Autodesk Inventor part; units mm, degrees
ref_plane "YZ Plane" through (0, 0, 0) normal (1, 0, 0) x (0, 1, 0)
ref_plane "XZ Plane" through (0, 0, 0) normal (0, 1, 0) x (-1, 0, 0)
ref_plane "XY Plane" through (0, 0, 0) normal (0, 0, 1) x (1, 0, 0)
sketch "Sketch7" plane through (0, 0, 0) normal (0, 1, 0) x (-1, 0, 0)
  circle A0 centre (0, 0) radius 25
  circle A1 centre (0, 0) radius 15
  dimension "d19" = 50
  dimension "d20" = 30
extrude "Extrusion5" add sketch "Sketch7" against normal blind 30 contours A1
extrude "Extrusion6" add sketch "Sketch7" along normal blind 200 contours A0 | A1
sketch "Sketch8" plane through (0, 0, 0) normal (1, 0, 0) x (0, 1, 0)
  line L0 (200, -25) -> (200, 25)
  line L1 (0, -25) -> (0, 25)
  line L2 (0, 25) -> (200, 25)
  line L3 (0, -25) -> (200, -25)
  line L4 (200, -25) -> (200, 25)
  line L5 (200, -25) -> (130, -25)
  line L6 (130, -25) -> (130, 25)
  line L7 (130, 25) -> (200, 25)
  line L8 (200, 25) -> (200, -25)
  circle A0 centre (175, 0) radius 25
  circle A1 centre (175, 0) radius 15
  point P0 (0, 0)
  point P1 (0, 0)
  point P2 (175, -25)
  point P3 (175, 25)
  dimension "d25" = 70
  dimension "d26" = 50
  dimension "d27" = 30
extrude "Extrusion7" cut sketch "Sketch8" along normal mid plane 200 contours L3 A0 L0 | A0 L2 L0 | A0 | L3 L6 L2 A0 | A1
extrude "Extrusion8" add sketch "Sketch8" along normal mid plane 20 contours A0 | L3 L6 L2 A0
properties part number "Manipulator Link Type 2"
Work out the finished part from the listing and answer in its coordinate system (mm). A direction names the side the tool comes from. Give positions to 0.01 mm unless a question says otherwise; leave off trailing zeros. Order: outer loops, then holes, each group sorted by start corner. A loop starts at its lowest first (then second) coordinate and runs counter-clockwise, first axis right, second up. Notation, with made-up numbers: (49, -1.5) -> (103, -1.5) arc R32 cw to (103, 31.5) -> close; hole circle Ø2 at (12.25, -14.5). An arc over 180 degrees is marked (long way). One line per item, written item: value.
Item 1: Determine the mould class of faces 5 (the flat face through (-16, 130, 0)), 6 (the cylindrical face through (-0.14, 160.015, -0.66)), 7 (the cylindrical face through (14.985, -14.79, 0.66)), 8 (the flat face through (0, 152, 25)) for opening direction Z: released by +Z, released by -Z, zero draft, split by the parting line, or undercut.
Answer sheet:
face 5: zero draft
face 6: undercut
face 7: split by the parting line
face 8: released by +Z
Item 2: Flat-ended cylindrical pins translate along their axes: P1, Ø4, axis at x = 13, z = 16.5, coming from the -Y side; P2, Ø4, axis at y = 157, z = -14, coming from the -X side; P3, Ø4, axis at y = -1.5, z = 6, coming from the +X side; P4, Ø15, axis at y = 172.5, z = -5.5, coming from the -X side. Find the tip coordinate at first contact, or state that the pin passes through.
Answer sheet:
P1: y = 0
P2: x = -10
P3: x = 24.56
P4: through
Item 3: A tool of negligible diameter and unlimited length cuts with its end or side. For faces 1 (the flat face through (-10, 157, 0)), 2 (the flat face through (0, 152, -25)), 3 (the cylindrical face through (-23.846, 64.09, -7.509)), 4 (the flat face through (10, 157, 0)), from which of +Z, -Z, +X, -X, +Y, -Y can it reach the whole face along a straight path? Write none if from no direction.
Answer sheet:
face 1: +Z, -Z, -X, +Y
face 2: -Z, +X, -X, +Y, -Y
face 3: -Y
face 4: +Z, -Z, +X, +Y
Item 4: Straight lines are drawn through the part: probe 1 along Z at (x, y) = (-1.75, 175); probe 2 along Y at (x, z) = (20, 3); probe 3 along X at (y, z) = (131, -16.5). For each, find the intervals that lie inside material, in ascending order.
Answer sheet:
probe 1: -25 to -15, 15 to 25
probe 2: 0 to 130
probe 3: -10 to 10
Item 5: Find section C-C, the plane z = -18. Give the vertices of the cut face in (x, y), plus the area to 3 significant figures.
Answer sheet:
outline: (-17.35, 0) -> (17.35, 0) -> (17.35, 130) -> (10, 130) -> (10, 192.35) -> (-10, 192.35) -> (-10, 130) -> (-17.35, 130) -> close
area: 5,760 mm²
Item 6: Find section B-B, the plane x = -8. Give the vertices of the cut face in (y, z).
Answer sheet:
outline: (-30, -12.69) -> (0, -12.69) -> (0, -23.69) -> (130, -23.69) -> (130, -25) -> (175, -25) arc R25 ccw to (175, 25) -> (130, 25) -> (130, 23.69) -> (0, 23.69) -> (0, 12.69) -> (-30, 12.69) -> close; hole circle Ø30 at (175, 0)
Item 7: Find section D-D, the plane y = 146. Give the vertices of the cut face in (x, z).
Answer sheet:
outline: (-10, -25) -> (10, -25) -> (10, 25) -> (-10, 25) -> close
Item 8: Find section A-A, the plane z = 0. Give the vertices of the cut face in (x, y).
Answer sheet:
outline: (-25, 0) -> (-15, 0) -> (-15, -30) -> (15, -30) -> (15, 0) -> (25, 0) -> (25, 130) -> (10, 130) -> (10, 160) -> (-10, 160) -> (-10, 130) -> (-25, 130) -> close; (-10, 190) -> (10, 190) -> (10, 200) -> (-10, 200) -> close
